Autodesk Inventor part; units mm, degrees
ref_plane "YZ Plane" through (0, 0, 0) normal (1, 0, 0) x (0, 1, 0)
ref_plane "XZ Plane" through (0, 0, 0) normal (0, 1, 0) x (-1, 0, 0)
ref_plane "XY Plane" through (0, 0, 0) normal (0, 0, 1) x (1, 0, 0)
sketch "Sketch1" plane through (0, 0, 0) normal (0, 1, 0) x (-1, 0, 0)
  line L0 (0, 0) -> (11, 0)
  line L1 (11, 0) -> (11, -6)
  line L2 (11, -6) -> (0, -6)
  line L3 (0, -6) -> (0, 0)
  line L4 (0, 0) -> (-5, 0)
  line L5 (-5, 0) -> (-5, 12)
  line L6 (-5, 12) -> (0, 12)
  line L7 (0, 12) -> (0, 0)
  line L8 (0, -6) -> (-5, -6)
  line L9 (-5, -6) -> (-5, -18)
  line L10 (-5, -18) -> (0, -18)
  line L11 (0, -18) -> (0, -6)
  line L12 (-5, -6) -> (-45, -6)
  line L13 (-45, -6) -> (-45, 0)
  line L14 (-45, 0) -> (-5, 0)
  line L15 (-5, 0) -> (-5, -6)
  line L16 (-5, -6) -> (-45, -6)
  line L17 (-45, -6) -> (-45, -11)
  line L18 (-45, -11) -> (-5, -11)
  line L19 (-5, -11) -> (-5, -6)
  line L20 (-5, 0) -> (-45, 0)
  line L21 (-45, 0) -> (-45, 5)
  line L22 (-45, 5) -> (-5, 5)
  line L23 (-5, 5) -> (-5, 0)
  line L24 (-5, 0) -> (-10, 0)
  line L25 (-10, 0) -> (-10, 12)
  line L26 (-10, 12) -> (-5, 12)
  line L27 (-5, 12) -> (-5, 0)
  line L28 (0, 0) -> (5, 0)
  line L29 (5, 0) -> (5, 12)
  line L30 (5, 12) -> (0, 12)
  line L31 (0, 12) -> (0, 0)
  line L32 (0, -6) -> (5, -6)
  line L33 (5, -6) -> (5, -18)
  line L34 (5, -18) -> (0, -18)
  line L35 (0, -18) -> (0, -6)
  line L36 (-5, -18) -> (-10, -18)
  line L37 (-10, -18) -> (-10, -6)
  line L38 (-10, -6) -> (-5, -6)
  line L39 (-5, -6) -> (-5, -18)
  line L40 (11, 0) -> (5, 0)
  line L41 (5, 0) -> (5, 5)
  line L42 (5, 5) -> (11, 5)
  line L43 (11, 5) -> (11, 0)
  line L44 (11, -6) -> (5, -6)
  line L45 (5, -6) -> (5, -11)
  line L46 (5, -11) -> (11, -11)
  line L47 (11, -11) -> (11, -6)
  point P0 (-10, -11)
  point P1 (-10, 5)
  dimension "d0" = 11
  dimension "d1" = 6
  dimension "d2" = 5
  dimension "d3" = 12
  dimension "d4" = 5
  dimension "d5" = 12
  dimension "d6" = 40
  dimension "d7" = 5
  dimension "d8" = 5
  dimension "d9" = 5
  dimension "d10" = 5
  dimension "d11" = 5
  dimension "d12" = 5
extrude "Extrusion1" add sketch "Sketch1" along normal blind 5 contours L7 L30 L29 L0 | L29 L42 L43 L0 | L2 L33 L34 L11 | L14 L25 L22 L5 | L2 L47 L46 L33 | L9 L18 L37 L12 | L22 L25 L26 L5 | L14 L21 L22 L25 | L9 L36 L37 L18 | L37 L18 L17 L12
sketch "Sketch2" plane through (0, 5, 0) normal (0, 1, 0) x (1, 0, 0)
  line L0 (-11, 6) -> (0, 6)
  line L1 (0, 6) -> (0, 18)
  line L2 (0, 18) -> (-5, 18)
  line L3 (-5, 18) -> (-5, 11)
  line L4 (-5, 11) -> (-11, 11)
  line L5 (-11, 11) -> (-11, 6)
  line L6 (5, 6) -> (45, 6)
  line L7 (45, 6) -> (45, 11)
  line L8 (45, 11) -> (10, 11)
  line L9 (10, 11) -> (10, 18)
  line L10 (10, 18) -> (5, 18)
  line L11 (5, 18) -> (5, 6)
  line L12 (10, -12) -> (10, -5)
  line L13 (10, -5) -> (45, -5)
  line L14 (45, -5) -> (45, 0)
  line L15 (45, 0) -> (5, 0)
  line L16 (5, 0) -> (5, -12)
  line L17 (5, -12) -> (10, -12)
  line L18 (-11, -5) -> (-5, -5)
  line L19 (-5, -5) -> (-5, -12)
  line L20 (-5, -12) -> (0, -12)
  line L21 (0, -12) -> (0, 0)
  line L22 (0, 0) -> (-11, 0)
  line L23 (-11, 0) -> (-11, -5)
  line L24 (-11, 11) -> (10, 11)
  line L25 (10, 11) -> (10, -5)
  line L26 (10, -5) -> (-11, -5)
  line L27 (-11, -5) -> (-11, 11)
  line L28 (-5, 18) -> (10, 18)
  line L29 (10, 18) -> (10, 11)
  line L30 (10, 11) -> (-5, 11)
  line L31 (-5, 11) -> (-5, 18)
  line L32 (-5, -5) -> (10, -5)
  line L33 (10, -5) -> (10, -12)
  line L34 (10, -12) -> (-5, -12)
  line L35 (-5, -12) -> (-5, -5)
extrude "Extrusion2" add sketch "Sketch2" along normal blind 5 contours L5 L4 L24 L1 L0 | L0 L1 L24 L11 L6 L25 L15 L16 L26 L21 L22 L27 | L22 L21 L26 L18 L23 | L24 L3 L2 L1 | L1 L28 L11 L24 | L24 L25 L6 L11 | L11 L10 L9 L24 | L26 L16 L34 L21 | L21 L20 L19 L26 | L26 L12 L17 L16 | L16 L15 L25 L26
sketch "Sketch3" plane through (0, 5, 0) normal (0, 1, 0) x (1, 0, 0)
  point P0 (0, 0)
sketch "Sketch4" plane through (0, 5, 0) normal (0, 1, 0) x (1, 0, 0)
  line L0 (10, 0) -> (10, -5)
  line L1 (10, -5) -> (45, -5)
  line L2 (45, -5) -> (45, 0)
  line L3 (45, 0) -> (10, 0)
  line L4 (10, 11) -> (10, 6)
  line L5 (10, 6) -> (45, 6)
  line L6 (45, 6) -> (45, 11)
  line L7 (45, 11) -> (10, 11)
  point P0 (0, 0)
extrude "Extrusion3" add sketch "Sketch4" along normal blind 5
sketch "Sketch5" plane through (5, 0, -6) normal (0, 0, 1) x (1, 0, 0)
  line L0 (40, 0) -> (40, 10)
  line L1 (40, 0) -> (40, 10)
  line L2 (0, 0) -> (40, 0)
  line L3 (40, 0) -> (40, 10)
  line L4 (5, 10) -> (40, 10)
  line L5 (5, 5) -> (5, 10)
  line L6 (0, 5) -> (5, 5)
  line L7 (0, 0) -> (0, 5)
  line L8 (40, 10) -> (5, 10)
  line L9 (5, 10) -> (5, 5)
  line L10 (5, 5) -> (40, 5)
  line L11 (40, 5) -> (40, 10)
  point P0 (-5, 0)
  dimension "d19" = 5
extrude "Extrusion4" add sketch "Sketch5" along normal up to surface (6 mm away) contours L10 L5 L4 L0
properties part number "BTArm"
The listing builds one solid part. Answer for the finished solid, in the listing's coordinates (mm). A direction names the side the tool comes from. Coordinates: 2 decimals unless noted, no trailing zeros. Loops run counter-clockwise (first coordinate to the right, second up) from the corner with the lowest first, then second, coordinate; pieces in that order, holes last. Notation, with made-up numbers: M -10,71 L 49,71 A11 cw 49,91 Z; hole C 77.25,-19 d1. An arc over 180 degrees is marked long. Answer in a Markdown table with one row per item.
1) Find section A-A (y = 2.25). Determine the outline of the cut face in (x, z), then the cut area to 3 significant figures.
Answers below:
| item | result |
|---|---|
| outline | M -11,-11 L -5,-11 L -5,-18 L 0,-18 L 0,-6 L -11,-6 Z; M -11,0 L 0,0 L 0,12 L -5,12 L -5,5 L -11,5 Z; M 5,-18 L 10,-18 L 10,-11 L 45,-11 L 45,-6 L 5,-6 Z; M 5,0 L 45,0 L 45,5 L 10,5 L 10,12 L 5,12 Z |
| area | 650 mm^2 |
2) Find section B-B (x = 33). Determine the outline of the cut face in (y, z), then the cut area to 3 significant figures.
Answers below:
| item | result |
|---|---|
| outline | M 0,-11 L 10,-11 L 10,5 L 0,5 L 0,0 L 5,0 L 5,-6 L 0,-6 Z |
| area | 130 mm^2 |
3) Which of the six approach directions +Z, -Z, +X, -X, +Y, -Y give full straight-line access (tool end or side, diameter ignored) to faces 1 (the flat face through (25, 2, -6)), 2 (the flat face through (5, 2, -12)), 3 (the flat face through (-5, 5, -15)), 4 (the flat face through (3, 6, -18)), 5 (the flat face through (-5, 5, 8))?
Answers below:
| item | result |
|---|---|
| face 1 | +X, -X, -Y |
| face 2 | +Z, -Z, -Y |
| face 3 | -Z, -X, +Y, -Y |
| face 4 | -Z, +X, -X, +Y, -Y |
| face 5 | +Z, -X, +Y, -Y |
4) Determine the mould class of faces 6 (the flat face through (-8, 5, -11)), 7 (the flat face through (-6, 2, -6)), 8 (the flat face through (-4, 0, -11)), 9 (the flat face through (-5, 2, 0)) for opening direction Z: released by +Z, released by -Z, zero draft, split by the parting line, or undercut.
Answers below:
| item | result |
|---|---|
| face 6 | released by -Z |
| face 7 | undercut |
| face 8 | zero draft |
| face 9 | undercut |
5) Find section C-C (z = -9.5). Determine the outline of the cut face in (x, y).
Answers below:
| item | result |
|---|---|
| outline | M -11,0 L 0,0 L 0,5 L 5,5 L 5,0 L 45,0 L 45,10 L -11,10 Z |
6) Given pin 1 (2 mm diameter, centred on y = 5, z = 8, fed in from +X); pin 2 (5 mm diameter, centred on x = -9.5, y = 6, fed in from -Z); pin 3 (3 mm diameter, centred on x = 20.5, y = 7, fed in from +Z); pin 4 (8 mm diameter, centred on x = 14.5, z = 0.5, fed in from -Y), each flat-ended and moving along its own axis, determine where each tip first touches the part or whether it passes through.
Answers below:
| item | result |
|---|---|
| pin 1 | x = 10 |
| pin 2 | z = -11 |
| pin 3 | z = 5 |
| pin 4 | y = 0 |
7) Find section D-D (y = 9). Determine the outline of the cut face in (x, z), then the cut area to 3 significant figures.
Answers below:
| item | result |
|---|---|
| outline | M -11,-11 L -5,-11 L -5,-18 L 10,-18 L 10,-11 L 45,-11 L 45,5 L 10,5 L 10,12 L -5,12 L -5,5 L -11,5 Z |
| area | 1,110 mm^2 |
8) Find the intervals of material crossed by probe 1 along X at (y, z) = (4, -7.5); probe 2 along Z at (x, y) = (41.5, 1.25); probe 3 along Z at (x, y) = (-3, 1), in increasing order.
Answers below:
| item | result |
|---|---|
| probe 1 | -11 to 0, 5 to 45 |
| probe 2 | -11 to -6, 0 to 5 |
| probe 3 | -18 to -6, 0 to 12 |
